from build123d import *

# Parameters (mm, degrees)
F0_W     = 60
F0_H     = 20.3
F1_DEPTH = 1.6
F2_W     = 10
F2_H     = 1.9
F3_DEPTH = 25
F4_SIZE  = 0.5
F5_R     = 0.94999


# Not quite as in the source:
# - a fillet or chamfer is up to 0.001 mm smaller than in the source, because OpenCascade refuses the exact size


with BuildPart() as f1:
    # F0 (on Front) → F1 (new body)
    with BuildSketch(Plane.XZ):
        with Locations((19.8222492922, -0.2282736823)):
            Rectangle(F0_W, F0_H)
    extrude(amount=F1_DEPTH)

    # F2 (on Front) → F3 (cut)
    with BuildSketch(Plane.XZ):
        with Locations((-6.7777507078, -2.2282736823)):
            Rectangle(F2_W, F2_H)
    extrude(amount=F3_DEPTH, mode=Mode.SUBTRACT)

    # F4
    f4_edges = [f1.edges().sort_by_distance(p)[0] for p in [
        (-10.177751, -0.8, 9.921726),
        (-10.177751, -0.8, -1.278274),
        (-10.177751, -0.8, -3.178274),
        (-10.177751, -0.8, -10.378274),
    ]]
    chamfer(f4_edges, length=F4_SIZE)

    # F5 (radius 0.95 in the source; OpenCascade refuses exactly that, so slightly less here)
    f5_edges = [f1.edges().sort_by_distance(p)[0] for p in [
        (-1.777751, -0.8, -1.278274),
        (-1.777751, -0.8, -3.178274),
    ]]
    fillet(f5_edges, radius=F5_R)


solid = f1.part
The listing builds one solid part. Answer for the finished solid, in the listing's coordinates (mm). A direction names the side the tool comes from. Round coordinates to 2 decimals unless told otherwise and drop trailing zeros. Write item = value, one per line. Start each with the question number.
1) For faces 1 (the flat face through (-6, -1, -1.278)), 2 (the flat face through (19, -1.6, 0)), determine the directions among +Z, -Z, +X, -X, +Y, -Y from which every point of the face is accessible in a straight line to the end or side of a thin tool.
2) For a pull along Z with two mould halves and no side action, classify faces 3 (the flat face through (20, -1, 9.922)), 4 (the flat face through (-6, -1, -3.178)), 5 (the flat face through (19, 0, 0)), 6 (the flat face through (20, -1, -10.378)) as released by +Z, released by -Z, zero draft, split by the parting line, or undercut.
3) Straight lines are drawn through the part: L1, parallel to Z at x = -6, y = -0.6; L2, parallel to X at y = -0.45, z = -3.25; L3, parallel to X at y = -0.4, z = -1. For each, find the intervals that lie inside material, in ascending order.
Results list:
q1.face_1 = -X, +Y, -Y
q1.face_2 = +Z, -Z, +X, -X, -Y
q2.face_3 = released by +Z
q2.face_4 = undercut
q2.face_5 = zero draft
q2.face_6 = released by -Z
q3.L1 = -10.38 to -3.18, -1.28 to 9.92
q3.L2 = -9.75 to 49.82
q3.L3 = -9.96 to 49.82
